Input: part model. Units: mm. Frame: model coordinates. A direction names the side the tool comes from. Give positions to 0.01 mm unless a question says otherwise; leave off trailing zeros. Order: outer loops, then holes, each group sorted by start corner. A loop starts at its lowest first (then second) coordinate and runs counter-clockwise, first axis right, second up. Notation, with made-up numbers: (9.25, 5) -> (57.25, 5) arc R18 cw to (57.25, 18) -> close; hole circle Ø4 at (65.25, 24). An arc over 180 degrees is marked (long way). Use a Markdown table: item, result. Add a question column.
Autodesk Inventor part; units mm, degrees
ref_plane "YZ Plane" through (0, 0, 0) normal (1, 0, 0) x (0, 1, 0)
ref_plane "XZ Plane" through (0, 0, 0) normal (0, 1, 0) x (-1, 0, 0)
ref_plane "XY Plane" through (0, 0, 0) normal (0, 0, 1) x (1, 0, 0)
sketch "Skizze1" plane through (0, 0, 0) normal (1, 0, 0) x (0, 1, 0)
  line L0 (0, 0) -> (28, 0)
  line L1 (28, 0) -> (28, -50)
  line L2 (28, -50) -> (0, -50)
  line L3 (0, -50) -> (0, 0)
  dimension "d0" = 50
  dimension "d1" = 28
extrude "Extrusion1" add sketch "Skizze1" along normal blind 2
sketch "Skizze2" plane through (2, 0, 0) normal (1, 0, 0) x (0, 0, -1)
  line L0 (2.2, 25.8) -> (47.8, 25.8)
  line L1 (47.8, 25.8) -> (47.8, 2.2)
  line L2 (47.8, 2.2) -> (2.2, 2.2)
  line L3 (2.2, 2.2) -> (2.2, 25.8)
  line L4 (0, 28) -> (0, 0)
  line L5 (0, 0) -> (50, 0)
  dimension "d4" = 45.6
  dimension "d5" = 23.6
  dimension "d6" = 2.2
  dimension "d7" = 2.2
extrude "Extrusion2" add sketch "Skizze2" along normal blind 1.5
chamfer "Fase1" distance 0.5 angle 45 4 edges at (3.5, 2.2, -25) (3.5, 14, -2.2) (3.5, 14, -47.8) (3.5, 25.8, -25)
sketch "Skizze3" plane through (0, 0, 0) normal (-1, 0, 0) x (0, 0, 1)
  line L0 (-50, 0) -> (-50, 28)
  line L1 (-50, 9) -> (-60, 9)
  line L2 (-60, 9) -> (-60, 19)
  line L3 (-60, 19) -> (-50, 19)
  line L4 (-50, 19) -> (-50, 9)
  line L5 (-50, 28) -> (0, 28)
  line L6 (-30, 28) -> (-20, 28)
  line L7 (-20, 28) -> (-20, 38)
  line L8 (-20, 38) -> (-30, 38)
  line L9 (-30, 38) -> (-30, 28)
  line L10 (-30, 0) -> (-20, 0)
  line L11 (-20, 0) -> (-20, -10)
  line L12 (-20, -10) -> (-30, -10)
  line L13 (-30, -10) -> (-30, 0)
  line L14 (0, 28) -> (0, 0)
  line L15 (0, 9) -> (10, 9)
  line L16 (10, 9) -> (10, 19)
  line L17 (10, 19) -> (0, 19)
  line L18 (0, 19) -> (0, 9)
  line L19 (0, 0) -> (-50, 0)
  point P0 (0, 19)
  dimension "d13" = 10
  dimension "d14" = 10
  dimension "d15" = 10
  dimension "d16" = 10
  dimension "d17" = 10
  dimension "d18" = 10
  dimension "d19" = 10
  dimension "d20" = 10
  dimension "d21" = 20
  dimension "d22" = 20
  dimension "d23" = 9
  dimension "d24" = 9
extrude "Extrusion3" add sketch "Skizze3" against normal blind 2 contours L1 L2 L3 L0 | L10 L11 L12 L13 | L9 L8 L7 L5 | L14 L17 L16 L15
fillet "Rundung1" radius 2 16 edges at (1, 28, -30) (1, 38, -30) (1, 38, -20) (1, 19, -50) (1, 19, -60) (1, 9, -60) (1, 19, 10) (1, -10, -30) (1, 9, -50) (1, -10, -20) (1, 9, 10) (1, 0, -20) (1, 9, 0) (1, 19, 0) (1, 28, -20) (1, 0, -30)
sketch "Skizze4" plane through (0, 0, 0) normal (-1, 0, 0) x (0, 0, 1)
  circle A0 centre (-25, 34) radius 2.75
  circle A1 centre (6, 14) radius 2.75
  circle A2 centre (-25, -6) radius 2.75
  circle A3 centre (-56, 14) radius 2.75
  line L0 (-30, 36) -> (-30, 30)
  line L1 (-52, 19) -> (-58, 19)
  line L2 (8, 19) -> (2, 19)
  line L3 (-30, -2) -> (-30, -8)
  line L4 (10, 11) -> (10, 17)
  line L5 (-28, -10) -> (-22, -10)
  line L6 (-60, 17) -> (-60, 11)
  line L7 (-22, 38) -> (-28, 38)
  point P0 (0, 0)
  dimension "d28" = 5.5
  dimension "d29" = 5
  dimension "d30" = 5
  dimension "d31" = 5
  dimension "d32" = 5
  dimension "d33" = 4
  dimension "d34" = 4
  dimension "d35" = 4
  dimension "d36" = 4
extrude "Extrusion4" cut sketch "Skizze4" against normal blind 2
properties part number "gehaeuse_deckel"
Q1. Section query D-D (z = -15). Return loops of the section in (x, y).
Q2. Access query for faces 1 (the flat face through (1, 14, -60)), 2 (the flat face through (1, 19, 5)), 3 (the flat face through (1, -5, -20)), 4 (the flat face through (1, 33, -30)), 5 (the cylindrical face through (1.01, -0.57, -30.6)). Directions: +Z, -Z, +X, -X, +Y, -Y. A direction counts if a zero-diameter tool reaches every point of the face in a straight line with its end or side. Return the directions, or none.
Q3. First-contact query: pin 1 (1.5 mm diameter, centred on x = 3, z = -42, fed in from +Y); pin 2 (2 mm diameter, centred on x = 0.5, y = 5, fed in from +Z); pin 3 (1.6 mm diameter, centred on x = 0.5, z = -54, fed in from -Y); pin 4 (5 mm diameter, centred on y = 14, z = -56, fed in from +X). Flat tips, straight axial feed; report the tip coordinate or a pass-through.
Q4. Ray query, line 1 (Y direction, x = 1.25, z = -25); line 2 (Y direction, x = 1.2, z = 6); line 3 (Y direction, x = 2.3, z = -21). Return the intervals inside material, ascending.
Q5. Section query C-C (y = -6). Return loops of the section in (x, z), plus the area to 3 significant figures.
Q6. Section query B-B (y = 14). Return loops of the section in (x, z), plus the area to 3 significant figures.
Q7. Section query A-A (z = -56). Return loops of the section in (x, y).
Solution:
| question | item | result |
|---|---|---|
| 1 | outline | (0, 0) -> (2, 0) -> (2, 2.2) -> (3, 2.2) -> (3.5, 2.7) -> (3.5, 25.3) -> (3, 25.8) -> (2, 25.8) -> (2, 28) -> (0, 28) -> close |
| 2 | face 1 | -Z, +X, -X, +Y, -Y |
| 2 | face 2 | +Z, +X, -X, +Y |
| 2 | face 3 | +Z, +X, -X, -Y |
| 2 | face 4 | -Z, +X, -X, +Y |
| 2 | face 5 | -Z, +X, -X, -Y |
| 3 | pin 1 | stops at y = 25.8 |
| 3 | pin 2 | stops at z = 0 |
| 3 | pin 3 | stops at y = 9 |
| 3 | pin 4 | passes through |
| 4 | line 1 | y = -10 to -8.75, -3.25 to 31.25, 36.75 to 38 |
| 4 | line 2 | y = 9 to 11.25, 16.75 to 19 |
| 4 | line 3 | y = 2.2 to 25.8 |
| 5 | outline | (0, -30) -> (2, -30) -> (2, -27.75) -> (0, -27.75) -> close; (0, -22.25) -> (2, -22.25) -> (2, -20) -> (0, -20) -> close |
| 5 | area | 9.00 mm² |
| 6 | outline | (0, -60) -> (2, -60) -> (2, -58.75) -> (0, -58.75) -> close; (0, -53.25) -> (2, -53.25) -> (2, -47.8) -> (3, -47.8) -> (3.5, -47.3) -> (3.5, -2.7) -> (3, -2.2) -> (2, -2.2) -> (2, 3.25) -> (0, 3.25) -> close; (0, 8.75) -> (2, 8.75) -> (2, 10) -> (0, 10) -> close |
| 6 | area | 186 mm² |
| 7 | outline | (0, 9) -> (2, 9) -> (2, 11.25) -> (0, 11.25) -> close; (0, 16.75) -> (2, 16.75) -> (2, 19) -> (0, 19) -> close |
